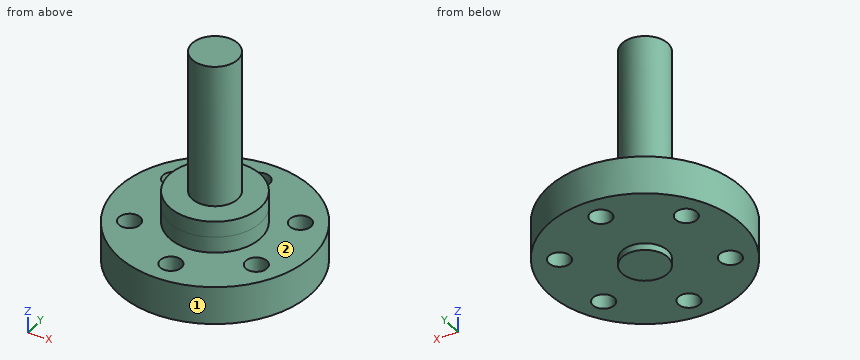
from build123d import *

# Parameters (mm, degrees)
SKETCH1_R           = 3
BOSS_EXTRUDE1_DEPTH = 29
SKETCH2_R           = 6
BOSS_EXTRUDE2_DEPTH = 2.1
SKETCH3_R           = 12.7
BOSS_EXTRUDE3_DEPTH = 5
SKETCH4_R           = 6
BOSS_EXTRUDE4_DEPTH = 2.1
SKETCH10_R          = 1.4
CUT_EXTRUDE1_DEPTH  = 5


with BuildPart() as part:
    # Sketch1 → Boss-Extrude1 (new body)
    with BuildSketch(Plane.XY):
        Circle(SKETCH1_R)
    extrude(amount=BOSS_EXTRUDE1_DEPTH)

    # Sketch2 → Boss-Extrude2 (add)
    with BuildSketch(Plane.XY.offset(8)):
        Circle(SKETCH2_R)
    extrude(amount=-BOSS_EXTRUDE2_DEPTH)

    # Sketch3 → Boss-Extrude3 (add)
    with BuildSketch(Plane(origin=(0, 0, 5.9), x_dir=(-1, 0, 0), z_dir=(0, 0, -1))):
        Circle(SKETCH3_R)
    extrude(amount=BOSS_EXTRUDE3_DEPTH)

    # Sketch4 → Boss-Extrude4 (add)
    with BuildSketch(Plane.XY.offset(8)):
        Circle(SKETCH4_R)
    extrude(amount=BOSS_EXTRUDE4_DEPTH)

    # Sketch10 → Cut-Extrude1 (cut)
    with BuildSketch(Plane(origin=(0, 0, 0.9), x_dir=(-1, 0, 0), z_dir=(0, 0, -1))):
        with Locations((8.227241336, 4.75)):
            Circle(SKETCH10_R)
        with Locations((0, 9.5)):
            Circle(SKETCH10_R)
        with Locations((8.227241336, -4.75)):
            Circle(SKETCH10_R)
        with Locations((0, -9.5)):
            Circle(SKETCH10_R)
        with Locations((-8.227241336, -4.75)):
            Circle(SKETCH10_R)
        with Locations((-8.227241336, 4.75)):
            Circle(SKETCH10_R)
    extrude(amount=-CUT_EXTRUDE1_DEPTH, mode=Mode.SUBTRACT)


solid = part.part
Design review of the part built by this model. Coordinates are the model's own, in mm. Face numbers are marked on the shaded views. A direction names the side the tool comes from. Round coordinates to 2 decimals unless told otherwise and drop trailing zeros. Write each loop counter-clockwise with the first axis right and the second up, starting at its lowest first coordinate (ties: lowest second). Pieces come first, ordered by that corner, then holes. Notation, with made-up numbers: (52, 40.5) - (109, 40.5) arc R24 cw to (109, 63.5) - close; hole circle Ø5 at (83, 53). An arc over 180 degrees is marked (long way). Use a Markdown table: item, result. Add a question column.
1. We need section C-C (y = 9.5). State the section outline as (x, z) points.
2. We need section D-D (x = 7.5). State the section outline as (y, z) points.
3. Clearance check with flat-ended pins moving along their axes: pin 1 (1.7 mm diameter, centred on x = -8.23, y = 4.75, fed in from -Z); pin 2 (2 mm diameter, centred on x = -3.5, z = 20, fed in from -Y); pin 3 (1 mm diameter, centred on y = 0.5, z = 26, fed in from -X); pin 4 (8 mm diameter, centred on x = -9, z = 5, fed in from +Y). State where each tip first meets the part, or that it passes through.
4. We need section B-B (y = -4.75). State the section outline as (x, z) points, then the cut area to 3 significant figures.
5. For the marked faces 1 and 2, list the 3-axis set-ups (+Z, -Z, +X, -X, +Y, -Y) from which the entire face can be reached by the end or side of a thin tool; tool diameter is ignored.
6. We need section A-A (x = 0). State the section outline as (y, z) points.
7. Wall thickness on probe 1 along X at (y, z) = (3.75, 5.25); probe 2 along Z at (x, y) = (-5, 7.25); probe 3 along Z at (x, y) = (-1.75, -3): over which ranges is each line inside the solid? List them lowest first.
Output:
| question | item | result |
|---|---|---|
| 1 | outline | (-8.43, 0.9) - (-1.4, 0.9) - (-1.4, 5.9) - (-8.43, 5.9) - close; (1.4, 0.9) - (8.43, 0.9) - (8.43, 5.9) - (1.4, 5.9) - close |
| 2 | outline | (-10.25, 0.9) - (-5.95, 0.9) - (-5.95, 5.9) - (-10.25, 5.9) - close; (-3.55, 0.9) - (3.55, 0.9) - (3.55, 5.9) - (-3.55, 5.9) - close; (5.95, 0.9) - (10.25, 0.9) - (10.25, 5.9) - (5.95, 5.9) - close |
| 3 | pin 1 | passes through |
| 3 | pin 2 | stops at y = -1.66 |
| 3 | pin 3 | stops at x = -3 |
| 3 | pin 4 | stops at y = 11.67 |
| 4 | outline | (-11.78, 0.9) - (-9.63, 0.9) - (-9.63, 5.9) - (-11.78, 5.9) - close; (-6.83, 0.9) - (6.83, 0.9) - (6.83, 5.9) - (3.67, 5.9) - (3.67, 10.1) - (-3.67, 10.1) - (-3.67, 5.9) - (-6.83, 5.9) - close; (9.63, 0.9) - (11.78, 0.9) - (11.78, 5.9) - (9.63, 5.9) - close |
| 4 | area | 121 mm2 |
| 5 | face 1 | +Z, -Z |
| 5 | face 2 | +Z |
| 6 | outline | (-12.7, 0.9) - (-10.9, 0.9) - (-10.9, 5.9) - (-12.7, 5.9) - close; (-8.1, 0.9) - (-3, 0.9) - (-3, 0) - (3, 0) - (3, 0.9) - (8.1, 0.9) - (8.1, 5.9) - (6, 5.9) - (6, 10.1) - (3, 10.1) - (3, 29) - (-3, 29) - (-3, 10.1) - (-6, 10.1) - (-6, 5.9) - (-8.1, 5.9) - close; (10.9, 0.9) - (12.7, 0.9) - (12.7, 5.9) - (10.9, 5.9) - close |
| 7 | probe 1 | x = -12.13 to -9.21, -7.25 to 7.25, 9.21 to 12.13 |
| 7 | probe 2 | z = 0.9 to 5.9 |
| 7 | probe 3 | z = 0.9 to 10.1 |
